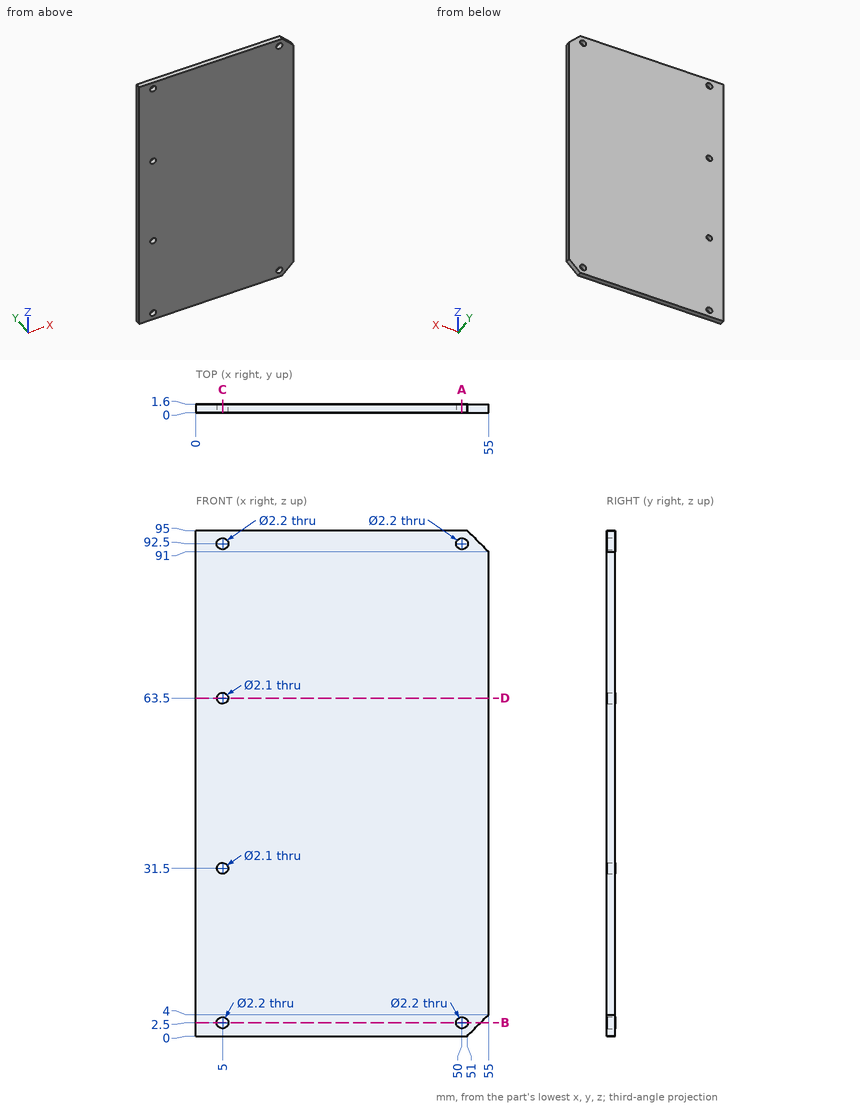
Verification items for this drawing (mm, ordinates from the low corner). Give positions to 0.01 mm unless a question says otherwise; leave off trailing zeros. Loops run counter-clockwise (first coordinate to the right, second up) from the corner with the lowest first, then second, coordinate; pieces in that order, holes last.
1. Cross-section at B-B on z = 2.5. Record the cut outline in (x, y).
Derived:
outline: (0, 0) - (3.9, 0) - (3.9, 1.6) - (0, 1.6) - close; (6.1, 0) - (48.9, 0) - (48.9, 1.6) - (6.1, 1.6) - close; (51.1, 0) - (53.5, 0) - (53.5, 1.6) - (51.1, 1.6) - close
2. Material ranges on probe 1 along Z at (x, y) = (5, 0.7); probe 2 along Z at (x, y) = (50, 1); probe 3 along Z at (x, y) = (50.5, 1.15), recorded low to high.
Derived:
probe 1: z = 0 to 1.4, 3.6 to 30.45, 32.55 to 62.45, 64.55 to 91.4, 93.6 to 95
probe 2: z = 0 to 1.4, 3.6 to 91.4, 93.6 to 95
probe 3: z = 0 to 1.52, 3.48 to 91.52, 93.48 to 95
3. Cross-section at A-A on x = 50. Record the cut outline in (y, z), and give its area (3 significant figures).
Derived:
outline: (0, 0) - (1.6, 0) - (1.6, 1.4) - (0, 1.4) - close; (0, 3.6) - (1.6, 3.6) - (1.6, 91.4) - (0, 91.4) - close; (0, 93.6) - (1.6, 93.6) - (1.6, 95) - (0, 95) - close
area: 145 mm2
4. Cross-section at C-C on x = 5. Record the cut outline in (y, z).
Derived:
outline: (0, 0) - (1.6, 0) - (1.6, 1.4) - (0, 1.4) - close; (0, 3.6) - (1.6, 3.6) - (1.6, 30.45) - (0, 30.45) - close; (0, 32.55) - (1.6, 32.55) - (1.6, 62.45) - (0, 62.45) - close; (0, 64.55) - (1.6, 64.55) - (1.6, 91.4) - (0, 91.4) - close; (0, 93.6) - (1.6, 93.6) - (1.6, 95) - (0, 95) - close
5. Cross-section at D-D on z = 63.5. Record the cut outline in (x, y).
Derived:
outline: (0, 0) - (3.95, 0) - (3.95, 1.6) - (0, 1.6) - close; (6.05, 0) - (55, 0) - (55, 1.6) - (6.05, 1.6) - close
